Read the model definition and answer for the solid it produces. Units are mm, in the model's axes. A direction names the side the tool comes from. Coordinates: 2 decimals unless noted, no trailing zeros. Write each loop counter-clockwise with the first axis right and the second up, starting at its lowest first coordinate (ties: lowest second). Pieces come first, ordered by that corner, then holes.
Item 1: Section B-B (x = 0) is taken. Give the vertices of the cut face in (y, z).
Item 2: Section D-D (x = 8) is taken. Give the vertices of the cut face in (y, z).
Item 3: Determine the mould class of faces 5 (the face through (-9.76, 16.48, -2.17)), 6 (the face through (26.78, 7.4, -29.71)), 7 (the face through (2.51, 7, -39)) for opening direction Z: released by +Z, released by -Z, zero draft, split by the parting line, or undercut.
Item 4: Straight lines are drawn through the part: probe 1 along Y at (x, z) = (10.5, 35.5); probe 2 along Z at (x, y) = (0, 9); probe 3 along X at (y, z) = (7.5, 0). For each, find the intervals that lie inside material, in ascending order.
Item 5: Section A-A (z = 0) is taken. Give the vertices of the cut face in (x, y), then the cut area to 4 significant figures.
Item 6: Each of these flat-tipped pins is pushed along its axis until it touches: P1, Ø16, axis at x = 0, z = 0, coming from the +Y side; P2, Ø2.5, axis at y = 9.5, z = -38.5, coming from the -X side; P3, Ø8, axis at x = -22.5, y = 9, coming from the -Z side; P4, Ø3, axis at x = 0, z = 0, coming from the +Y side. Where does it stop, or does it pass through?
Item 7: A tool of negligible diameter and unlimited length cuts with its end or side. For faces 1 (the face through (36.02, 7.395, 14.343)), 2 (the face through (-39.12, 7.4, -8.34)), 3 (the face through (15.281, 7.395, 34.236)), 4 (the face through (34.76, 7.4, -17.17)), from which of +Z, -Z, +X, -X, +Y, -Y can it reach the whole face along a straight path? Write none if from no direction.
Item 8: Section C-C (y = -1.25) is taken. Give the vertices of the cut face in (x, z).
from build123d import *

# Parameters (mm, degrees)
CROQUIS1_R                   = 40
SALIENTE_EXTRUIR1_DEPTH      = 15
CORTAR_EXTRUIR1_START        = -16
CROQUIS2_W                   = 5.020915278
CROQUIS2_H                   = 5.016516428
CORTAR_EXTRUIR1_DEPTH        = 68
MATRIZC1_COUNT               = 30
SALIENTE_EXTRUIR2_DEPTH      = 18
SALIENTE_EXTRUIR2_DEPTH_BACK = 3
CROQUIS3_R                   = 12.5
CROQUIS3_R_2                 = 10
CORTAR_EXTRUIR2_DEPTH        = 60
CORTAR_EXTRUIR2_DEPTH_BACK   = 27
CROQUIS4_R                   = 2.5


with BuildPart() as part:
    # Croquis1 → Saliente-Extruir1 (new body)
    with BuildSketch(Plane(origin=(0, 0, 0), x_dir=(1, 0, 0), z_dir=(0, 1, 0))):
        with Locations(Location((0, 0, 0), (0, 0, 270))):
            Circle(CROQUIS1_R)
    extrude(amount=SALIENTE_EXTRUIR1_DEPTH)

    # Croquis2 → Cortar-Extruir1 (cut)
    with BuildSketch(Plane(origin=(0, 0, 0), x_dir=(1, 0, 0), z_dir=(0, 1, 0)).offset(CORTAR_EXTRUIR1_START)):
        with Locations((0, 40)):
            Rectangle(CROQUIS2_W, CROQUIS2_H)
    cortar_extruir1 = extrude(amount=CORTAR_EXTRUIR1_DEPTH, mode=Mode.SUBTRACT)

    # MatrizC1: Cortar-Extruir1 ×30 about axis
    matrizc1_axis = Axis((0, 0, 0), (0, 1, 0))
    for i in range(1, MATRIZC1_COUNT):
        add(cortar_extruir1.rotate(matrizc1_axis, i * 360 / MATRIZC1_COUNT), mode=Mode.SUBTRACT)

    # Croquis3 → Saliente-Extruir2 (add, two sides: drawn at the far end of the back side and taken through both)
    with BuildSketch(Plane(origin=(0, 0, 0), x_dir=(1, 0, 0), z_dir=(0, 1, 0)).offset(-SALIENTE_EXTRUIR2_DEPTH_BACK)):
        with Locations(Location((0, 0, 0), (0, 0, 270))):
            Circle(CROQUIS3_R)
        with Locations(Location((0, 0, 0), (0, 0, 270))):
            Circle(CROQUIS3_R_2, mode=Mode.SUBTRACT)
    extrude(amount=SALIENTE_EXTRUIR2_DEPTH + SALIENTE_EXTRUIR2_DEPTH_BACK)

    # Croquis4 → Cortar-Extruir2 (cut, two sides: drawn at the far end of the back side and taken through both)
    with BuildSketch(Plane(origin=(0, 0, 0), x_dir=(1, 0, 0), z_dir=(0, 1, 0)).offset(-CORTAR_EXTRUIR2_DEPTH_BACK)):
        with Locations(Location((0, 0, 0), (0, 0, 270))):
            Circle(CROQUIS4_R)
    extrude(amount=CORTAR_EXTRUIR2_DEPTH + CORTAR_EXTRUIR2_DEPTH_BACK, mode=Mode.SUBTRACT)


solid = part.part
Established:
1. outline: (-3, -12.5) - (0, -12.5) - (0, -37.49) - (15, -37.49) - (15, -12.5) - (18, -12.5) - (18, -10) - (15, -10) - (15, -2.5) - (0, -2.5) - (0, -10) - (-3, -10) - close; (-3, 10) - (0, 10) - (0, 2.5) - (15, 2.5) - (15, 10) - (18, 10) - (18, 12.5) - (15, 12.5) - (15, 37.49) - (0, 37.49) - (0, 12.5) - (-3, 12.5) - close
2. outline: (-3, -9.6) - (0, -9.6) - (0, -36.63) - (15, -36.63) - (15, -9.6) - (18, -9.6) - (18, -6) - (15, -6) - (15, 6) - (18, 6) - (18, 9.6) - (15, 9.6) - (15, 36.63) - (0, 36.63) - (0, 9.6) - (-3, 9.6) - (-3, 6) - (0, 6) - (0, -6) - (-3, -6) - close
3. face 5: undercut
3. face 6: released by -Z
3. face 7: zero draft
4. probe 1: y = 0 to 15
4. probe 2: z = -37.49 to -2.5, 2.5 to 37.49
4. probe 3: x = -40 to -2.5, 2.5 to 40
5. outline: (-40, 0) - (-12.5, 0) - (-12.5, -3) - (-10, -3) - (-10, 0) - (-2.5, 0) - (-2.5, 15) - (-10, 15) - (-10, 18) - (-12.5, 18) - (-12.5, 15) - (-40, 15) - close; (2.5, 0) - (10, 0) - (10, -3) - (12.5, -3) - (12.5, 0) - (40, 0) - (40, 15) - (12.5, 15) - (12.5, 18) - (10, 18) - (10, 15) - (2.5, 15) - close
5. area: 1,155 mm2
6. P1: stops at y = 15
6. P2: stops at x = -13.94
6. P3: stops at z = -35.45
6. P4: passes through
7. face 1: +X, +Y, -Y
7. face 2: -Z, -X, +Y, -Y
7. face 3: +Y, -Y
7. face 4: -Z, +Y, -Y
8. outline: circle Ø25 at (0, 0); hole circle Ø20 at (0, 0)
